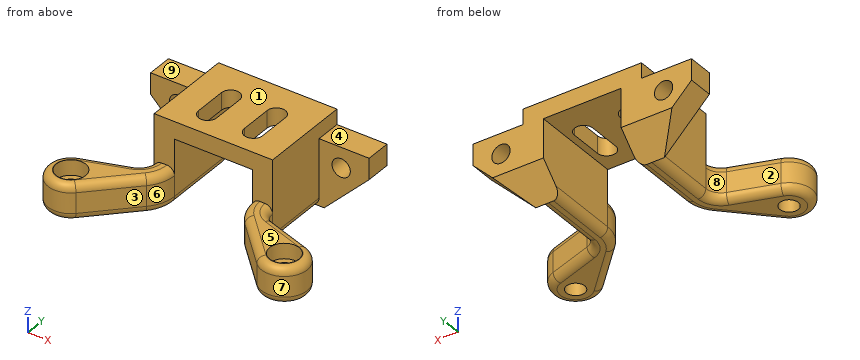
```python
from build123d import *

# Parameters (mm, degrees)
SKETCH_R        = 1.8
PAD_DEPTH       = 7
SKETCH001_R     = 2.9
POCKET_DEPTH    = 3
SKETCH002_W     = 9.85
SKETCH002_H     = 5
PAD001_DEPTH    = 6
SKETCH005_R     = 1.8
POCKET002_DEPTH = 5
SKETCH003_W     = 23.3
SKETCH003_H     = 18
PAD002_DEPTH    = 9
SKETCH004_W     = 15.3
SKETCH004_H     = 18
POCKET001_DEPTH = 12.6
POCKET003_DEPTH = 47.001
POCKET004_DEPTH = 5
POCKET005_DEPTH = 16.001
FILLET_R        = 1.5


with BuildPart() as part:
    # Sketch → Pad (new body)
    with BuildSketch(Plane.XY):
        with BuildLine():
            Line((-21.5, 0), (-21.5, -5))
            Line((-21.5, -5), (-11.65, -5))
            Line((-11.65, -5), (-11.65, -18))
            ThreePointArc((-13.707898, -20.848235), (-12.218302, -19.756942), (-11.65, -18))
            Line((-13.707898, -20.848235), (-22.413154, -23.727647))
            ThreePointArc((-22.413154, -23.727647), (-24.822377, -30.374749), (-17.795838, -31.159643))
            Line((-9.665748, -22.915), (-17.795838, -31.159643))
            ThreePointArc((-9.665748, -22.915), (-8.173513, -20.656147), (-7.65, -18))
            Line((-7.65, -18), (7.65, -18))
            ThreePointArc((7.65, -18), (8.173513, -20.656147), (9.665748, -22.915))
            Line((9.665748, -22.915), (17.795838, -31.159643))
            ThreePointArc((17.795838, -31.159643), (24.822377, -30.374749), (22.413154, -23.727647))
            Line((13.707898, -20.848235), (22.413154, -23.727647))
            ThreePointArc((11.65, -18), (12.218302, -19.756942), (13.707898, -20.848235))
            Line((11.65, -5), (11.65, -18))
            Line((21.5, -5), (11.65, -5))
            Line((21.5, -5), (21.5, 0))
            Line((21.5, 0), (-21.5, 0))
        make_face()
        with Locations((-21, -28)):
            Circle(SKETCH_R, mode=Mode.SUBTRACT)
        with Locations((21, -28)):
            Circle(SKETCH_R, mode=Mode.SUBTRACT)
    extrude(amount=PAD_DEPTH)

    # Sketch001 (on Face22 of Pad) → Pocket (cut)
    with BuildSketch(Plane.XY.offset(7)):
        with Locations((-21, -28)):
            Circle(SKETCH001_R)
        with Locations((21, -28)):
            Circle(SKETCH001_R)
    extrude(amount=-POCKET_DEPTH, mode=Mode.SUBTRACT)

    # Sketch002 (on Face5 of Pocket) → Pad001 (join)
    with BuildSketch(Plane.XY.offset(7)):
        with Locations((16.575, -2.5)):
            Rectangle(SKETCH002_W, SKETCH002_H)
        with Locations((-16.575, -2.5)):
            Rectangle(SKETCH002_W, SKETCH002_H)
    extrude(amount=PAD001_DEPTH)

    # Sketch005 (on Face29 of Pad001) → Pocket002 (cut)
    with BuildSketch(Plane(origin=(0, 0, 0), x_dir=(-1, 0, 0), z_dir=(0, 1, 0))):
        with Locations((-16, 9)):
            Circle(SKETCH005_R)
        with Locations((16, 9)):
            Circle(SKETCH005_R)
    extrude(amount=-POCKET002_DEPTH, mode=Mode.SUBTRACT)

    # Sketch003 (on Face3 of Pad001) → Pad002 (join)
    with BuildSketch(Plane.XY.offset(7)):
        with Locations((0, -9)):
            Rectangle(SKETCH003_W, SKETCH003_H)
    extrude(amount=PAD002_DEPTH)

    # Sketch004 (on Face1 of Pad002) → Pocket001 (cut)
    with BuildSketch(Plane(origin=(0, 0, 0), x_dir=(1, 0, 0), z_dir=(0, 0, -1))):
        with Locations((0, 9)):
            Rectangle(SKETCH004_W, SKETCH004_H)
    extrude(amount=-POCKET001_DEPTH, mode=Mode.SUBTRACT)

    # Sketch006 (on Face21 of Pocket001) → Pocket003 (cut, through all)
    with BuildSketch(Plane(origin=(-21.5, 0, 0), x_dir=(0, -1, 0), z_dir=(-1, 0, 0))):
        Polygon((5, 0), (0, 0), (0, 5), align=None)
    extrude(amount=-POCKET003_DEPTH, mode=Mode.SUBTRACT)

    # Sketch007 (on Face1 of Pocket003) → Pocket004 (cut)
    with BuildSketch(Plane.XZ.offset(5)):
        Polygon((-21.5, 0), (-21.5, 8.85), (-12.65, 0), align=None)
        Polygon((21.5, 0), (21.5, 8.85), (12.65, 0), align=None)
    extrude(amount=-POCKET004_DEPTH, mode=Mode.SUBTRACT)

    # Sketch008 (on Face11 of Pocket004) → Pocket005 (cut, through all)
    with BuildSketch(Plane.XY.offset(16)):
        with BuildLine():
            ThreePointArc((-2.7, -6.8), (-4.5, -5), (-6.3, -6.8))
            Line((-6.3, -6.8), (-6.3, -13.2))
            ThreePointArc((-6.3, -13.2), (-4.5, -15), (-2.7, -13.2))
            Line((-2.7, -6.8), (-2.7, -13.2))
        make_face()
        with BuildLine():
            ThreePointArc((6.3, -6.8), (4.5, -5), (2.7, -6.8))
            Line((2.7, -6.8), (2.7, -13.2))
            ThreePointArc((2.7, -13.2), (4.5, -15), (6.3, -13.2))
            Line((6.3, -6.8), (6.3, -13.2))
        make_face()
    extrude(amount=-POCKET005_DEPTH, mode=Mode.SUBTRACT)

    # Fillet
    fillet_edges = [part.edges().sort_by_distance(p)[0] for p in [
        (-7.65, -11.5, 0),
        (7.65, -11.5, 0),
        (-13.730793, -27.037322, 7),
        (13.730793, -27.037322, 7),
    ]]
    fillet(fillet_edges, radius=FILLET_R)


solid = part.part
```
Design review of the part built by this model. Coordinates are the model's own, in mm. Face numbers are marked on the shaded views. A direction names the side the tool comes from. Give positions to 0.01 mm unless a question says otherwise; leave off trailing zeros. Order: outer loops, then holes, each group sorted by start corner. A loop starts at its lowest first (then second) coordinate and runs counter-clockwise, first axis right, second up. Notation, with made-up numbers: (88.5, -9) - (127.5, -9) arc R20 cw to (127.5, -1) - close; hole circle Ø5 at (32.25, 26.5). An arc over 180 degrees is marked (long way). Use a Markdown table: item, result. Add a question column.
(1) Add section B-B on y = -6. Give the boundary of the cut face in (x, z).
(2) Clearance check with flat-ended pins moving along their axes: P1, Ø3, axis at x = -21, y = -28, coming from the +Z side; P2, Ø2, axis at y = -3, z = 11.5, coming from the -X side; P3, Ø2, axis at y = -14.5, z = 2.5, coming from the +X side; P4, Ø1.5, axis at x = -14, y = -23, coming from the +Z side. State where each tip first meets the part, or that it passes through.
(3) Machinability: for the marked faces 1, 2, 3, 4 and 5, which of the approach directions +Z, -Z, +X, -X, +Y, -Y give a long, thin tool a straight path to every point of the face, cutting with its end or side? Answer none if there is none.
(4) Mouldability with a two-part tool opening along Y and no side actions: class the marked faces 6, 7, 8 and 9 as +Y half, -Y half, draft (parallel to the pull), parting line (faces both ways), or undercut.
(5) Add section C-C on x = -16. Give the number of separate pieces and of enclosed holes in the cut face, then the cut area to 3 significant figures.
(6) Wall thickness on probe 1 along X at (y, z) = (-15.5, 2); probe 2 along X at (y, z) = (-28, 0.9); probe 3 along Y at (x, z) = (21, 6.1): over which ranges is each line inside the solid? List them lowest first. Write a range as [from, to].
(7) Add section A-A on x = 4.5. Give the boundary of the cut face in (y, z).
Report:
| question | item | result |
|---|---|---|
| 1 | outline | (-11.65, 1.5) arc R1.5 ccw to (-10.15, 0) - (-9.15, 0) arc R1.5 ccw to (-7.65, 1.5) - (-7.65, 12.6) - (-6.11, 12.6) - (-6.11, 16) - (-11.65, 16) - close; (-2.89, 12.6) - (2.89, 12.6) - (2.89, 16) - (-2.89, 16) - close; (6.11, 12.6) - (7.65, 12.6) - (7.65, 1.5) arc R1.5 ccw to (9.15, 0) - (10.15, 0) arc R1.5 ccw to (11.65, 1.5) - (11.65, 16) - (6.11, 16) - close |
| 2 | P1 | passes through |
| 2 | P2 | stops at x = -21.5 |
| 2 | P3 | stops at x = 11.65 |
| 2 | P4 | stops at z = 7 |
| 3 | face 1 | +Z, +X, -X, +Y, -Y |
| 3 | face 2 | +Z, -Z, -X |
| 3 | face 3 | +Z, -Z, -Y |
| 3 | face 4 | +Z, +X, +Y, -Y |
| 3 | face 5 | +Z, +X, -X, -Y |
| 4 | face 6 | -Y half |
| 4 | face 7 | parting line |
| 4 | face 8 | undercut |
| 4 | face 9 | draft |
| 5 | separate pieces | 3 |
| 5 | enclosed holes | 0 |
| 5 | area | 80.6 mm² |
| 6 | probe 1 | x = [-11.65, -7.65], [7.65, 11.65] |
| 6 | probe 2 | x = [-25.37, -22.8], [-19.2, -14.86], [14.86, 19.2], [22.8, 25.37] |
| 6 | probe 3 | y = [-32.37, -30.9], [-25.1, -23.39] |
| 7 | outline | (-18, 12.6) - (-15, 12.6) - (-15, 16) - (-18, 16) - close; (-5, 12.6) - (0, 12.6) - (0, 16) - (-5, 16) - close |
